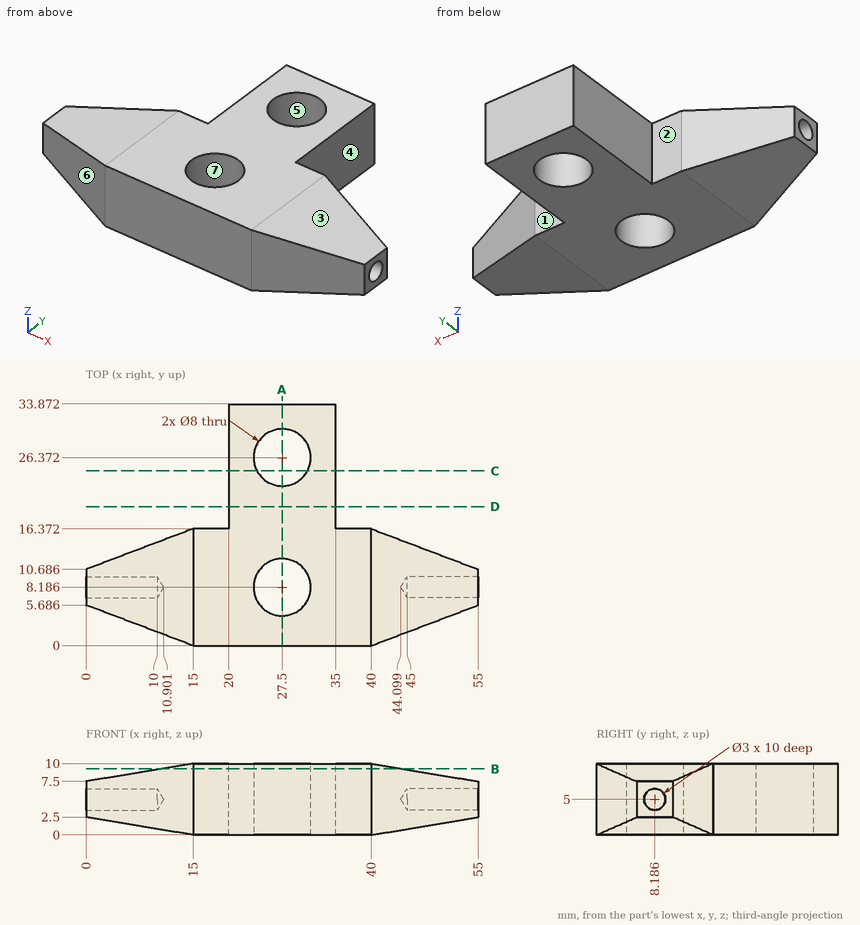
Input: dimensioned drawing with shaded views. Units: mm. Origin: part minimum x, y, z. A direction names the side the tool comes from. Give positions to 0.01 mm unless a question says otherwise; leave off trailing zeros. Loops run counter-clockwise (first coordinate to the right, second up) from the corner with the lowest first, then second, coordinate; pieces in that order, holes last. Notation, with made-up numbers: M -21.5,0 L 13.5,0 A19 cw 13.5,23 Z; hole C 68,75 d1. An arc over 180 degrees is marked long. Put each result on its own line as item: value.
1) Cut plane B-B, the plane z = 9.25. Return the cut outline in (x, y).
Computed values:
outline: M 10.5,1.71 L 15,0 L 40,0 L 44.5,1.71 L 44.5,14.67 L 40,16.37 L 35,16.37 L 35,33.87 L 20,33.87 L 20,16.37 L 15,16.37 L 10.5,14.67 Z; hole C 27.5,8.19 d8; hole C 27.5,26.37 d8
2) Cut plane A-A, the plane x = 27.5. Return the cut outline in (y, z).
Computed values:
outline: M 0,0 L 4.19,0 L 4.19,10 L 0,10 Z; M 12.19,0 L 22.37,0 L 22.37,10 L 12.19,10 Z; M 30.37,0 L 33.87,0 L 33.87,10 L 30.37,10 Z
3) Cut plane D-D, the plane y = 19.5. Return the cut outline in (x, z), plus the area to 3 significant figures.
Computed values:
outline: M 20,0 L 35,0 L 35,10 L 20,10 Z
area: 150 mm^2
4) Material intervals for L1, parallel to Y at x = 27.5, z = 5; L2, parallel to X at y = 8.5, z = 2.75; L3, parallel to X at y = 18.5, z = 3.5, sorted ascending. Write a range as from..to.
Computed values:
L1: y = 0..4.19, 12.19..22.37, 30.37..33.87
L2: x = 0..23.51, 31.49..55
L3: x = 20..35
5) Reachability of the marked faces 1, 2 and 3 from +Z, -Z, +X, -X, +Y, -Y: full face, straight path, thin tool, end or side. Return the list, or none.
Computed values:
face 1: +Z, -Z, +X, +Y
face 2: +Z, -Z, -X, +Y
face 3: +Z, +X, +Y, -Y
6) Cut plane C-C, the plane y = 24.5. Return the cut outline in (x, z) (1 decimal).
Computed values:
outline: M 20,0 L 24,0 L 24,10 L 20,10 Z; M 31,0 L 35,0 L 35,10 L 31,10 Z
7) Mould query, pull axis X, two halves, no side actions, for the marked faces 4, 5, 6 and 7. Classes: released by +X, released by -X, zero draft, split by the parting line, or undercut.
Computed values:
face 4: released by +X
face 5: undercut
face 6: released by -X
face 7: undercut
8) First-contact query: P1, Ø4, axis at y = 20.5, z = 2, coming from the +X side; P2, Ø2.5, axis at y = 8.19, z = 5, coming from the +X side; P3, Ø5, axis at y = 25, z = 4.5, coming from the -X side. Flat tips, straight axial feed; report the tip coordinate or a pass-through.
Computed values:
P1: stops at x = 35
P2: stops at x = 44.85
P3: stops at x = 20
